Here's how the part is built. I have some questions about the finished solid (model axes, mm). A direction names the side the tool comes from. Coordinates: 2 decimals unless noted, no trailing zeros. Order: outer loops, then holes, each group sorted by start corner. A loop starts at its lowest first (then second) coordinate and runs counter-clockwise, first axis right, second up. Notation, with made-up numbers: (31, 3.5) -> (44, 3.5) arc R23 ccw to (44, 22.5) -> close; hole circle Ø9 at (88, -9). An arc over 180 degrees is marked (long way). One line per item, written item: value. Start each with the question number.
```python
from build123d import *

# Parameters (mm, degrees)
F0_W     = 27
F0_H     = 5
F1_DEPTH = 40


with BuildPart() as f1:
    # F0 (on Top) → F1 (new body)
    with BuildSketch(Plane.XY):
        with BuildLine():
            Line((0, 30), (0, 0))
            Line((0, 0), (5, 0))
            Line((5, 0), (5, 16))
            ThreePointArc((5, 16), (9.100505, 25.899495), (19, 30))
            ThreePointArc((19, 30), (28.899495, 25.899495), (33, 16))
            Line((33, 16), (33, 0))
            Line((33, 0), (38, 0))
            Line((38, 0), (38, 30))
            ThreePointArc((38, 30), (33.606602, 40.606602), (23, 45))
            Line((23, 45), (15, 45))
            ThreePointArc((15, 45), (4.393398, 40.606602), (0, 30))
        make_face()
        with Locations((19, 35)):
            Rectangle(F0_W, F0_H, mode=Mode.SUBTRACT)
    extrude(amount=F1_DEPTH)


solid = f1.part
```
Q1. Imagine slicing it at B-B (y = 34.5). Write out the boundary of the cut face in (x, z).
Q2. Imagine slicing it at A-A (z = 24). Write out the boundary of the cut face in (x, y).
Q3. If we mould it in two halves opening along Y, with no side actions, what happens to faces 1 (the face through (19, 32.5, 20)), 2 (the face through (33.72, 40.49, 19.72)), 3 (the face through (0, 15, 20))? For each: +Y half, -Y half, draft (parallel to the pull), parting line (faces both ways), or undercut.
Q4. I need wall thicknesses on line 1 (X direction, y = 15.5, z = 16.5); line 2 (Y direction, x = 31, z = 15); line 3 (Y direction, x = 19, z = 3). Which ranges of each line are inside material? Lowest first, please.
Q5. Imagine slicing it at C-C (x = 25.5). Write out the boundary of the cut face in (y, z), plus the area to 3 significant figures.
Q6. Imagine slicing it at D-D (x = 3). Write out the boundary of the cut face in (y, z), plus the area to 3 significant figures.
Q7. For faces 4 (the face through (2, 0, 20)), 5 (the face through (33, 8, 20)), 6 (the face through (19, 37.5, 20)), which set-ups out of +Z, -Z, +X, -X, +Y, -Y let a thin tool reach every point of the face, with its end or its side?
Q8. For P1, Ø1.5, axis at y = 35, z = 12.5, coming from the +X side; P2, Ø5.5, axis at y = 35, z = 26, coming from the -X side; P3, Ø13.5, axis at x = 19, z = 20, coming from the -Y side, each with a flat end and sliding along its axis, tell me the tip position at first contact or that it passes through.
Completed:
1. outline: (0.69, 0) -> (5.5, 0) -> (5.5, 40) -> (0.69, 40) -> close; (32.5, 0) -> (37.31, 0) -> (37.31, 40) -> (32.5, 40) -> close
2. outline: (0, 0) -> (5, 0) -> (5, 16) arc R14 cw to (33, 16) -> (33, 0) -> (38, 0) -> (38, 30) arc R15 ccw to (23, 45) -> (15, 45) arc R15 ccw to (0, 30) -> close; hole (5.5, 32.5) -> (32.5, 32.5) -> (32.5, 37.5) -> (5.5, 37.5) -> close
3. face 1: undercut
3. face 2: +Y half
3. face 3: draft
4. line 1: x = 0 to 5, 33 to 38
4. line 2: y = 23.21 to 32.5, 37.5 to 42.69
4. line 3: y = 30 to 32.5, 37.5 to 45
5. outline: (28.4, 0) -> (32.5, 0) -> (32.5, 40) -> (28.4, 40) -> close; (37.5, 0) -> (44.79, 0) -> (44.79, 40) -> (37.5, 40) -> close
5. area: 456 mm2
6. outline: (0, 0) -> (39, 0) -> (39, 40) -> (0, 40) -> close
6. area: 1,560 mm2
7. face 4: +Z, -Z, +X, -X, -Y
7. face 5: +Z, -Z, -Y
7. face 6: +Z, -Z
8. P1: stops at x = 37.39
8. P2: stops at x = 0.17
8. P3: stops at y = 28.27
